from build123d import *

# Parameters (mm, degrees)
F0_W     = 125
F0_H     = 254
F1_DEPTH = 10.16
F2_R     = 5.07999


# Not quite as in the source:
# - a fillet or chamfer is up to 0.001 mm smaller than in the source, because OpenCascade refuses the exact size


with BuildPart() as f1:
    # F0 (on Top) → F1 (new body)
    with BuildSketch(Plane.XY):
        with Locations((0, 7.7496204972)):
            Rectangle(F0_W, F0_H)
        with BuildLine():
            ThreePointArc((12.9974298287, 0), (34.3412344545, -15.4252090897), (42.5, -40.4637716711))
            ThreePointArc((42.5, -40.4637716711), (-25.0385625813, -74.8050061256), (-12.9974298287, 0))
            Line((-12.9974298287, 0), (-13.0543755367, 0))
            Line((-13.0543755367, 0), (-13.0543755367, 76.8597647548))
            Line((-13.0543755367, 76.8597647548), (12.9974298287, 76.8597647548))
            Line((12.9974298287, 76.8597647548), (12.9974298287, 0))
        make_face(mode=Mode.SUBTRACT)
    extrude(amount=F1_DEPTH)

    # F2 (radius 5.08 in the source; OpenCascade refuses exactly that, so slightly less here)
    f2_edges = [f1.edges().sort_by_distance(p)[0] for p in [
        (0, 134.74962, 10.16),
        (-62.5, 134.74962, 5.08),
        (-62.5, 7.74962, 10.16),
        (62.5, 7.74962, 10.16),
        (0, -119.25038, 10.16),
        (-62.5, 7.74962, 0),
        (62.5, -119.25038, 5.08),
        (62.5, 134.74962, 5.08),
        (62.5, 7.74962, 0),
        (0, -119.25038, 0),
        (0, 134.74962, 0),
    ]]
    fillet(f2_edges, radius=F2_R)


solid = f1.part
Could you check a few things on this model? Use its own coordinates, in mm. A direction names the side the tool comes from. Coordinates: 2 decimals unless noted, no trailing zeros. Order: outer loops, then holes, each group sorted by start corner. A loop starts at its lowest first (then second) coordinate and runs counter-clockwise, first axis right, second up. Notation, with made-up numbers: (65, 26.25) -> (104, 26.25) arc R19 cw to (104, 50.25) -> close; hole circle Ø4 at (6, 41.5). An arc over 180 degrees is marked (long way). One line per item, written item: value. Start each with the question number.
1) We'd pull the mould along X, two halves only. Please class faces 3 (the cylindrical face through (61.051, 9.457, 8.632)), 4 (the cylindrical face through (1.68, -82.93, 5.01)), 5 (the cylindrical face through (0.804, 133.301, 8.632)): +X half, -X half, draft (parallel to the pull), parting line (faces both ways), or undercut.
2) Imagine slicing it at D-D on z = 7.75. List the corners of the cut face in (x, y) for me, plus the area to 3 significant figures.
3) If I drill on L1, parallel to Y at x = 0, z = 4.75; L2, parallel to X at y = 7, z = 5.25; L3, parallel to Y at x = 0, z = 7.75, over which ranges is the centre line in solid material (lowest first)? Write a range as [from, to].
4) I'm going to push flat-ended pins straight in: pin 1 (2 mm diameter, centred on x = -35.5, z = 8, fed in from -Y); pin 2 (5 mm diameter, centred on x = -18.5, z = 8, fed in from -Y); pin 3 (6 mm diameter, centred on x = -45.5, z = 1.5, fed in from +Y). Where does each tip first touch, or does it pass through?
5) Which directions (+Z, -Z, +X, -X, +Y, -Y) give clear straight access to the entire face, cutting with the end or side of a thin tool? Please do faces 1 (the cylindrical face through (-1.701, -117.802, 8.632)), 2 (the flat face through (-13.054, 38, 5)).
Answer list:
1. face 3: +X half
1. face 4: undercut
1. face 5: draft
2. outline: (-61.74, -118.49) -> (57.42, -118.49) arc R4.32 ccw to (61.74, -114.17) -> (61.74, 129.67) arc R4.32 ccw to (57.42, 133.99) -> (-57.42, 133.99) arc R4.32 ccw to (-61.74, 129.67) -> close; hole (-13.05, 0) -> (-13, 0) arc R42.5 ccw (long way) to (13, 0) -> (13, 76.86) -> (-13.05, 76.86) -> close
2. area: 23,500 mm2
3. L1: y = [-119.24, -82.96], [76.86, 134.74]
3. L2: x = [-62.5, -13.05], [13, 62.5]
3. L3: y = [-118.49, -82.96], [76.86, 133.99]
4. pin 1: stops at y = -118.87
4. pin 2: stops at y = -119.23
4. pin 3: stops at y = 134.72
5. face 1: +Z, +X, -X, -Y
5. face 2: +Z, -Z
